Autodesk Inventor part; units mm, degrees
ref_plane "YZ Plane" through (0, 0, 0) normal (1, 0, 0) x (0, 1, 0)
ref_plane "XZ Plane" through (0, 0, 0) normal (0, 1, 0) x (-1, 0, 0)
ref_plane "XY Plane" through (0, 0, 0) normal (0, 0, 1) x (1, 0, 0)
sketch "Sketch" plane through (0, 0, 0) normal (1, 0, 0) x (0, 1, 0)
  circle A0 centre (0, 0) radius 2.5
  dimension "d1" = 5
extrude "Body" add sketch "Sketch" along normal blind 30
chamfer "Chamfer1" distance 0.8 angle 15 1 edges at (0, -2.5, 0) measured on face at (20, 2.4919, -0.2012)
chamfer "Sketch2" distance 0.8 angle 15 1 edges at (30, -2.5, 0) measured on face at (20.2667, 2.4919, -0.2012)
equation "\"d1\" = NND"
equation "\"d2\" = NLG"
equation "\"d8\" = PHH"
equation "\"d9\" = FAWI"
equation "\"d12\" = PHH"
equation "\"d4\" = PHH"
equation "\"d5\" = FAWI"
equation "\"d11\" = PHH"
equation "\"NND\" = 5"
equation "\"NLG\" = 30"
equation "\"PHH\" = 0.8"
equation "\"FAWI\" = 15deg"
equation "\"PHH2\" = PHH"
equation "\"FAWI2\" = 15deg"
properties part number "ISO 8734 - 5 x 30 - A" material "Steel"
The model under review builds one solid part; all positions refer to its coordinate system, in mm. Coordinates: 2 decimals unless noted, no trailing zeros. Write each loop counter-clockwise with the first axis right and the second up, starting at its lowest first coordinate (ties: lowest second). Pieces come first, ordered by that corner, then holes. Notation, with made-up numbers: (-26, -6.75) - (-6, -6.75) arc R13 ccw to (-6, -2.75) - close; hole circle Ø3 at (6.25, 38.25). An arc over 180 degrees is marked (long way). Answer in a Markdown table with one row per item. Add a question column.
Q1. Consider section A-A on x = 4. Give the boundary of the cut face in (y, z), then the cut area to 3 significant figures.
Q2. Clearance check with a flat-ended pin moving along its axis: pin 1 (2 mm diameter, centred on x = 7.5, z = 0.5, fed in from -Y). State where the tip first meets the part, or that it passes through.
Q3. To check wall thickness, follow line 1 along Y through (x, z) = (8.75, 1); line 2 along Y through (x, z) = (9.25, 1.75); line 3 along Z through (x, y) = (7, 0.8). State the ranges of each line that lie inside material, in increasing order. Write a range as from..to.
Answers below:
| question | item | result |
|---|---|---|
| 1 | outline | circle Ø5 at (0, 0) |
| 1 | area | 19.6 mm² |
| 2 | pin 1 | y = -2.5 |
| 3 | line 1 | -2.29..2.29 |
| 3 | line 2 | -1.79..1.79 |
| 3 | line 3 | -2.37..2.37 |
